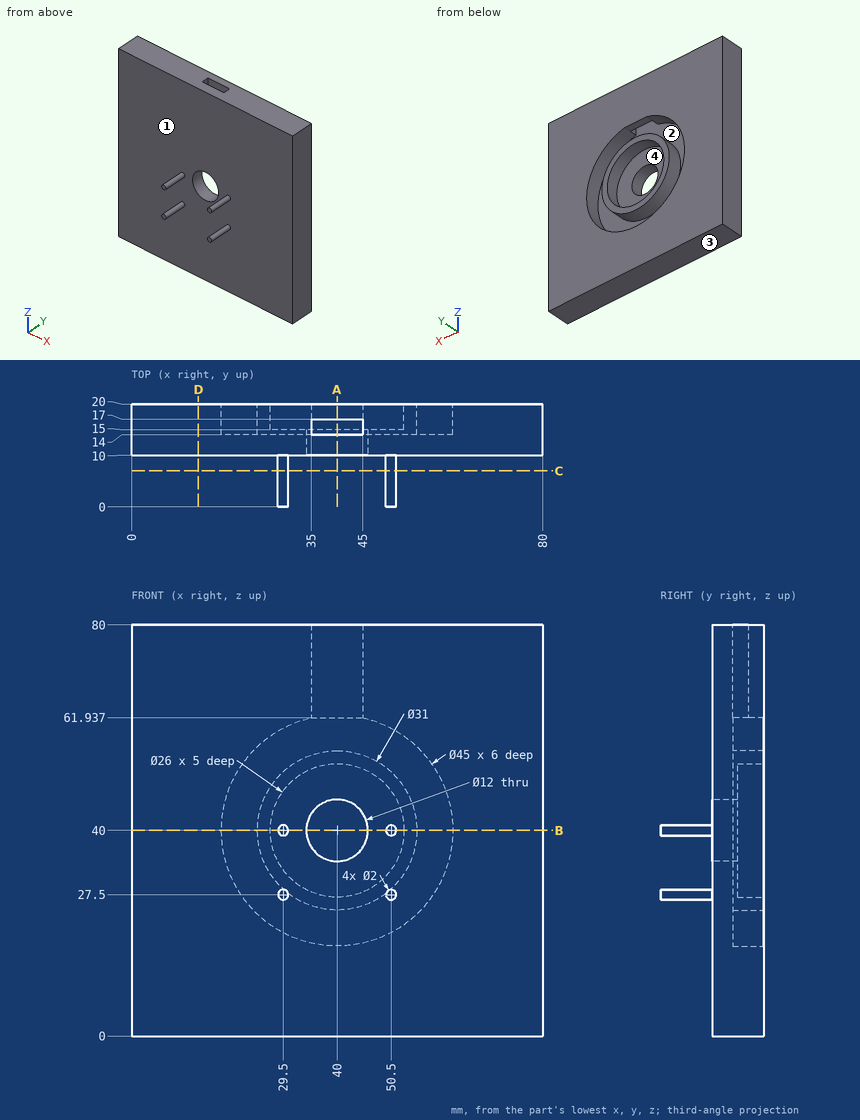
Part print with two shaded views. Sizes in mm from the minimum x, y, z corner. Coordinates: 2 decimals unless noted, no trailing zeros. Write each loop counter-clockwise with the first axis right and the second up, starting at its lowest first coordinate (ties: lowest second). Pieces come first, ordered by that corner, then holes. Notation, with made-up numbers: (10, 83.25) - (62, 83.25) arc R19 cw to (62, 87.25) - close; hole circle Ø4 at (69, 57). An arc over 180 degrees is marked (long way). Use a Markdown table: item, result. Add a question column.
Item 1: Two-plate mould, pull along Y, no slides. Class the marked faces 1, 2, 3 and 4: pulls with the +Y half, pulls with the -Y half, needs draft (parallel to the pull), parting line crosses it, or undercut.
Item 2: Drop flat-ended pins along their axis: pin 1 (8 mm diameter, centred on x = 37.5, z = 40, fed in from +Y); pin 2 (5 mm diameter, centred on x = 42, z = 72.5, fed in from -Y); pin 3 (2 mm diameter, centred on x = 68, y = 16.5, fed in from -Z); pin 4 (11 mm diameter, centred on x = 40, z = 40, fed in from -Y). Give the stop position or say it passes through.
Item 3: Band-saw the part on D-D, the plane x = 13. Write the cut outline in (y, z).
Item 4: Drill centre lines: line 1 along X through (y, z) = (17.25, 40); line 2 along X through (y, z) = (11, 40). Where is each one in solid material? Low to high.
Item 5: Band-saw the part on A-A, the plane x = 40. Write the cut outline in (y, z).
Item 6: Band-saw the part on B-B, the plane z = 40. Write the cut outline in (x, y).
Item 7: Band-saw the part on C-C, the plane y = 7. Write the cut outline in (x, z).
A:
| question | item | result |
|---|---|---|
| 1 | face 1 | pulls with the -Y half |
| 1 | face 2 | undercut |
| 1 | face 3 | needs draft |
| 1 | face 4 | pulls with the +Y half |
| 2 | pin 1 | stops at y = 15 |
| 2 | pin 2 | stops at y = 10 |
| 2 | pin 3 | stops at z = 0 |
| 2 | pin 4 | passes through |
| 3 | outline | (10, 0) - (20, 0) - (20, 80) - (10, 80) - close |
| 4 | line 1 | x = 0 to 17.5, 24.5 to 27, 53 to 55.5, 62.5 to 80 |
| 4 | line 2 | x = 0 to 34, 46 to 80 |
| 5 | outline | (10, 0) - (20, 0) - (20, 17.5) - (14, 17.5) - (14, 24.5) - (20, 24.5) - (20, 27) - (15, 27) - (15, 34) - (10, 34) - close; (10, 46) - (15, 46) - (15, 53) - (20, 53) - (20, 55.5) - (14, 55.5) - (14, 80) - (10, 80) - close; (17, 61.94) - (20, 61.94) - (20, 80) - (17, 80) - close |
| 6 | outline | (0, 10) - (28.5, 10) - (28.5, 0) - (30.5, 0) - (30.5, 10) - (34, 10) - (34, 15) - (27, 15) - (27, 20) - (24.5, 20) - (24.5, 14) - (17.5, 14) - (17.5, 20) - (0, 20) - close; (46, 10) - (49.5, 10) - (49.5, 0) - (51.5, 0) - (51.5, 10) - (80, 10) - (80, 20) - (62.5, 20) - (62.5, 14) - (55.5, 14) - (55.5, 20) - (53, 20) - (53, 15) - (46, 15) - close |
| 7 | outline | circle Ø2 at (29.5, 27.5); circle Ø2 at (29.5, 40); circle Ø2 at (50.5, 27.5); circle Ø2 at (50.5, 40) |
